```python
from build123d import *

# Parameters (mm, degrees)
F0_W     = 984.25
F0_H     = 1003.3
F0_W_2   = 127
F0_H_2   = 76.2
F1_DEPTH = 6.35
F2_DEPTH = 25.4
F3_DEPTH = 25.4


with BuildPart() as f1:
    # F0 (on Top) → F1 (new body)
    with BuildSketch(Plane.XY):
        with Locations((415.838617, 13.748734)):
            Rectangle(F0_W, F0_H)
        with Locations((415.838617, 375.698734)):
            Rectangle(F0_W_2, F0_H_2, mode=Mode.SUBTRACT)
    extrude(amount=F1_DEPTH)

    # F0 (on Top) → F2 (join)
    with BuildSketch(Plane.XY):
        with Locations((415.838617, 13.748734)):
            Rectangle(F0_W, F0_H)
        with Locations((415.838617, 375.698734)):
            Rectangle(F0_W_2, F0_H_2, mode=Mode.SUBTRACT)
    extrude(amount=F2_DEPTH)

    # F0 (on Top) → F3 (join)
    with BuildSketch(Plane.XY):
        with Locations((415.838617, 13.748734)):
            Rectangle(F0_W, F0_H)
        with Locations((415.838617, 375.698734)):
            Rectangle(F0_W_2, F0_H_2, mode=Mode.SUBTRACT)
    extrude(amount=F3_DEPTH)


solid = f1.part
```
The model under review builds one solid part; all positions refer to its coordinate system, in mm. A direction names the side the tool comes from. Round coordinates to 2 decimals unless told otherwise and drop trailing zeros. Loops run counter-clockwise (first coordinate to the right, second up) from the corner with the lowest first, then second, coordinate; pieces in that order, holes last. Notation, with made-up numbers: M 32.5,80.5 L 38.5,80.5 A22 cw 38.5,118.5 Z; hole C 9,80 d6. An arc over 180 degrees is marked long. Answer as a JSON object with one key per item and string values.
(1) Take a section at A-A on y = 398. Give the boundary of the cut face in (x, z).
Resolved:
{"outline": "M -76.29,0 L 352.34,0 L 352.34,25.4 L -76.29,25.4 Z; M 479.34,0 L 907.96,0 L 907.96,25.4 L 479.34,25.4 Z"}
(2) Draft analysis for pull direction Y (two halves, no side actions). For faces 1 (the flat face through (415, 337.599, 13)), 2 (the flat face through (409, -487.901, 13)), 3 (the flat face through (409, 21, 0)), state which applies: released by +Y, released by -Y, zero draft, split by the parting line, or undercut.
Resolved:
{"face 1": "undercut", "face 2": "released by -Y", "face 3": "zero draft"}
(3) Clearance check with a flat-ended pin moving along its axis: P1, Ø3, axis at x = 654, y = -370, coming from the -Z side. State where the tip first meets the part, or that it passes through.
Resolved:
{"P1": "z = 0"}
(4) Take a section at B-B on x = 406.5. Give the boundary of the cut face in (y, z), and give its area (3 significant figures).
Resolved:
{"outline": "M -487.9,0 L 337.6,0 L 337.6,25.4 L -487.9,25.4 Z; M 413.8,0 L 515.4,0 L 515.4,25.4 L 413.8,25.4 Z", "area": "23,500 mm²"}
(5) To check wall thickness, follow line 1 along Y through (x, z) = (424, 1.75). State the ranges of the line that lie inside material, in increasing order.
Resolved:
{"line 1": "-487.9 to 337.6, 413.8 to 515.4"}
(6) Tool access review of faces 4 (the flat face through (352.339, 375, 13)), 5 (the flat face through (907.964, 7, 13)): name each direction out of +Z, -Z, +X, -X, +Y, -Y from which nothing blocks a thin tool from reaching the whole face with its end or side.
Resolved:
{"face 4": "+Z, -Z", "face 5": "+Z, -Z, +X, +Y, -Y"}
